Geometry: final body of the model. Coordinates: model frame, mm. Coordinates: 2 decimals unless noted, no trailing zeros. Write each loop counter-clockwise with the first axis right and the second up, starting at its lowest first coordinate (ties: lowest second). Pieces come first, ordered by that corner, then holes. Notation, with made-up numbers: (44.5, -16) - (60.5, -16) arc R15 ccw to (60.5, 5) - close; hole circle Ø6 at (28.25, -36). An arc over 180 degrees is marked (long way). Answer as a JSON object with one key per item and string values. Group by question number.
Item 1: First-contact query: pin 1 Ø3 at (x, z) = (-63.5, 11.15) entering from -Y; pin 2 Ø3 at (x, y) = (-29, -4) entering from -Z; pin 3 Ø2 at (x, y) = (-1, -5.5) entering from -Z. Flat tips, straight axial feed; report the tip coordinate or a pass-through.
Item 2: Section A-A on x = 29.21. Return loops of the section in (y, z).
Item 3: Section D-D on y = -4. State how many separate pieces and enclosed holes the cut face has, and give its area (3 significant figures).
Item 4: Line query: line 1 along Z through (x, y) = (-38.1, -2.25); line 2 along Z through (x, y) = (-58, -3.5); line 3 along Z through (x, y) = (-63.5, -2.5). Output: solid intervals per line, ascending. Write a range as from..to.
Item 5: Section B-B on z = -12.7. Return loops of the section in (x, y).
Item 6: Mould query, pull axis Z, two halves, no side actions, for faces 1 (the flat face through (82.373, -3.131, 93.831)), 2 (the cylindrical face through (41.944, -3.131, -21.415)), 3 (the cylindrical face through (39.394, -3.131, 40.778)). Classes: pulls with the +Z half, pulls with the -Z half, needs draft (parallel to the pull), parting line crosses it, or undercut.
Item 7: Section C-C on x = -5.5. Return loops of the section in (y, z).
```python
from build123d import *

# Parameters (mm, degrees)
F0_R     = 2.5527
F0_R_2   = 14.2875
F0_R_3   = 4.7625
F0_R_4   = 11.1125
F1_DEPTH = 6.35


with BuildPart() as f1:
    # F0 (on Front) → F1 (new body)
    with BuildSketch(Plane.XZ):
        with BuildLine():
            Line((-99.147001, 36.428507), (-44.929465, -19.339581))
            ThreePointArc((-44.929465, -19.339581), (-41.990137, -21.394392), (-38.499317, -22.216626))
            Line((-38.499317, -22.216626), (-0.931741, -23.792961))
            ThreePointArc((-0.931741, -23.792961), (0, -23.8125), (0.931741, -23.792961))
            Line((0.931741, -23.792961), (38.499317, -22.216626))
            ThreePointArc((38.499317, -22.216626), (41.990137, -21.394392), (44.929465, -19.339581))
            Line((44.929465, -19.339581), (99.147001, 36.428507))
            ThreePointArc((99.147001, 36.428507), (108.088235, 61.457145), (95.037742, 84.610178))
            Line((95.037742, 84.610178), (69.349048, 103.313963))
            ThreePointArc((69.349048, 103.313963), (64.032071, 106.028196), (58.136106, 106.963559))
            Line((58.136106, 106.963559), (-58.136106, 106.963559))
            ThreePointArc((-58.136106, 106.963559), (-64.032071, 106.028196), (-69.349048, 103.313963))
            Line((-69.349048, 103.313963), (-95.037742, 84.610178))
            ThreePointArc((-95.037742, 84.610178), (-108.088235, 61.457145), (-99.147001, 36.428507))
        make_face()
        with Locations((-38.1, -12.7)):
            Circle(F0_R, mode=Mode.SUBTRACT)
        with Locations((-38.1, 0)):
            Circle(F0_R, mode=Mode.SUBTRACT)
        with Locations((0, -1.5875)):
            Circle(F0_R_2, mode=Mode.SUBTRACT)
        with Locations((-63.5, 11.149014)):
            Circle(F0_R, mode=Mode.SUBTRACT)
        with Locations((-58.239488, 40.776988)):
            Circle(F0_R, mode=Mode.SUBTRACT)
        with Locations((-38.1, 12.7)):
            Circle(F0_R, mode=Mode.SUBTRACT)
        with Locations((-41.275, 39.0525)):
            Circle(F0_R, mode=Mode.SUBTRACT)
        with Locations((38.1, -12.7)):
            Circle(F0_R, mode=Mode.SUBTRACT)
        with Locations((38.1, 0)):
            Circle(F0_R, mode=Mode.SUBTRACT)
        with Locations((38.1, 12.7)):
            Circle(F0_R, mode=Mode.SUBTRACT)
        with Locations((41.275, 39.0525)):
            Circle(F0_R, mode=Mode.SUBTRACT)
        with Locations((63.5, 11.149014)):
            Circle(F0_R, mode=Mode.SUBTRACT)
        with Locations((-76.2, 58.7375)):
            Circle(F0_R_3, mode=Mode.SUBTRACT)
        with Locations((0, 69.5325)):
            Circle(F0_R_2, mode=Mode.SUBTRACT)
        with Locations((-58.136106, 87.913559)):
            Circle(F0_R_4, mode=Mode.SUBTRACT)
        with Locations((-29.21, 100.613559)):
            Circle(F0_R, mode=Mode.SUBTRACT)
        with Locations((76.2, 58.7375)):
            Circle(F0_R_3, mode=Mode.SUBTRACT)
        with Locations((29.21, 100.613559)):
            Circle(F0_R, mode=Mode.SUBTRACT)
        with Locations((58.136106, 87.913559)):
            Circle(F0_R_4, mode=Mode.SUBTRACT)
    extrude(amount=F1_DEPTH)


solid = f1.part
```
Checks:
{
 "1": {"pin 1": "through", "pin 2": "z = -22.68", "pin 3": "z = -23.81"},
 "2": {"outline": "(-6.35, -22.61) - (0, -22.61) - (0, 98.06) - (-6.35, 98.06) - close; (-6.35, 103.17) - (0, 103.17) - (0, 106.96) - (-6.35, 106.96) - close"},
 "3": {"separate pieces": "1", "enclosed holes": "19", "area": "19,500 mm^2"},
 "4": {"line 1": "-22.23..-15.25, -10.15..-2.55, 2.55..10.15, 15.25..106.96", "line 2": "-5.9..38.24, 43.32..76.8, 99.03..106.96", "line 3": "-0.24..8.6, 13.7..78.18, 97.65..106.19"},
 "5": {"outline": "(-51.38, -6.35) - (-40.65, -6.35) - (-40.65, 0) - (-51.38, 0) - close; (-35.55, -6.35) - (-8.98, -6.35) - (-8.98, 0) - (-35.55, 0) - close; (8.98, -6.35) - (35.55, -6.35) - (35.55, 0) - (8.98, 0) - close; (40.65, -6.35) - (51.38, -6.35) - (51.38, 0) - (40.65, 0) - close"},
 "6": {"face 1": "pulls with the +Z half", "face 2": "pulls with the -Z half", "face 3": "undercut"},
 "7": {"outline": "(-6.35, -23.6) - (0, -23.6) - (0, -14.77) - (-6.35, -14.77) - close; (-6.35, 11.6) - (0, 11.6) - (0, 56.35) - (-6.35, 56.35) - close; (-6.35, 82.72) - (0, 82.72) - (0, 106.96) - (-6.35, 106.96) - close"}
}
